from build123d import *

# Parameters (mm, degrees)
F1_DEPTH = 67.4566328526
F2_DEPTH = 6.2197912484
F4_DEPTH = 12.4627631158


with BuildPart() as f1:
    # F0 (on Right) → F1 (new body)
    with BuildSketch(Plane.YZ):
        Polygon((-5.8088302612, 34.2432931066), (0, 34.2432931066), (0, -34.2432931066), (-5.8088302612, -34.2432931066), (-5.8088302612, -37.9646643996), (76.7590999603, -37.9646643996), (76.7590999603, 37.9646643996), (-5.8088302612, 37.9646643996), align=None)
    extrude(amount=F1_DEPTH)

    # F2 (add): a face of the model
    f2_faces = [f1.faces().sort_by_distance(p)[0] for p in [
        (33.7283164263, 76.7590999603, 0),
    ]]
    extrude(f2_faces, amount=F2_DEPTH)

    # F3 (on face) → F4 (join)
    with BuildSketch(Plane(origin=(0, 82.9788912088, 0), x_dir=(-1, 0, 0), z_dir=(0, 1, 0))):
        with BuildLine():
            ThreePointArc((-38.3854716222, 0.9479600765), (-36.6591605512, 5.8587284108), (-37.6652367413, 10.9659396112))
            ThreePointArc((-37.6652367413, 10.9659396112), (-40.901393767, 22.4123427927), (-52.0788472287, 18.3432652315))
            ThreePointArc((-52.0788472287, 18.3432652315), (-65.9917417473, 22.0669934876), (-55.7989236075, 11.8914716641))
            Line((-55.7989236075, 11.8914716641), (-55.7989236075, 0))
            Line((-55.7989236075, 0), (-50.582356751, 6.5680034459))
            Line((-50.582356751, 6.5680034459), (-46.5246960521, 6.5680034459))
            ThreePointArc((-46.5246960521, 6.5680034459), (-44.599657899, 1.9303920858), (-44.8609884943, -3.0840787076))
            Line((-44.8609884943, -3.0840787076), (-38.3854716222, 0.9479600765))
        make_face()
    extrude(amount=F4_DEPTH)


solid = f1.part
Design review of the part built by this model. Coordinates are the model's own, in mm. A direction names the side the tool comes from. Round coordinates to 2 decimals unless told otherwise and drop trailing zeros. Write each loop counter-clockwise with the first axis right and the second up, starting at its lowest first coordinate (ties: lowest second). Pieces come first, ordered by that corner, then holes. Notation, with made-up numbers: M -12,61.5 L 36,61.5 A19 ccw 36,80.5 Z; hole C -39.5,12 d2. An arc over 180 degrees is marked long. One line per item, written item: value. Start each with the question number.
1. Take a section at C-C on z = -9. State the section outline as (x, y) points, then the cut area to 3 significant figures.
2. Draft analysis for pull direction Z (two halves, no side actions). For faces 5 (the face through (33, 0, 0)), 6 (the face through (55.799, 89, 6)), 7 (the face through (33, 38, -37.965)), 8 (the face through (33, -3, -34.243)), state which applies: pulls with the +Z half, pulls with the -Z half, needs draft (parallel to the pull), parting line crosses it, or undercut.
3. Take a section at A-A on x = 30.5. State the section outline as (y, z) points.
4. To check wall thickness, follow probe 1 along Y at (x, z) = (28, 31); probe 2 along Y at (x, z) = (59, 21); probe 3 along Z at (x, y) = (47, 86). State the ranges of each line that lie inside material, in increasing order. Write a range as from..to.
5. Clearance check with flat-ended pins moving along their axes: P1, Ø2, axis at x = 35.5, z = 1.5, coming from the +Y side; P2, Ø9.5, axis at y = 90.5, z = 4.5, coming from the +X side; P3, Ø5, axis at x = 56.5, z = 9, coming from the -Y side. State where each tip first meets the part, or that it passes through.
6. Take a section at B-B on y = 88. State the section outline as (x, z) points, then the cut area to 3 significant figures.
7. Take a section at D-D on x = 48.5. State the section outline as (y, z) points.
8. For faces 1 (the face through (36.665, 89.123, 5.785)), 2 (the face through (41.669, 89.123, -1.096)), 3 (the face through (44.61, 89.12, 2)), 4 (the face through (49, 89, 6.568)), list the 3-axis set-ups (+Z, -Z, +X, -X, +Y, -Y) from which the entire face can be reached by the end or side of a thin tool; tool diameter is ignored.
Computed:
1. outline: M 0,0 L 67.46,0 L 67.46,82.98 L 0,82.98 Z
1. area: 5,600 mm²
2. face 5: undercut
2. face 6: needs draft
2. face 7: pulls with the -Z half
2. face 8: undercut
3. outline: M -5.81,-37.96 L 82.98,-37.96 L 82.98,37.96 L -5.81,37.96 L -5.81,34.24 L 0,34.24 L 0,-34.24 L -5.81,-34.24 Z
4. probe 1: y = 0..82.98
4. probe 2: y = 0..95.44
4. probe 3: z = 6.57..22.94
5. P1: stops at y = 82.98
5. P2: stops at x = 55.8
5. P3: stops at y = 0
6. outline: M 37.67,10.97 A9.89 ccw 38.39,0.95 L 44.86,-3.08 A11.36 cw 46.52,6.57 L 50.58,6.57 L 55.8,0 L 55.8,11.89 A7.45 ccw long 52.08,18.34 A8.12 ccw long Z
6. area: 508 mm²
7. outline: M -5.81,-37.96 L 82.98,-37.96 L 82.98,6.57 L 95.44,6.57 L 95.44,22.31 L 82.98,22.31 L 82.98,37.96 L -5.81,37.96 L -5.81,34.24 L 0,34.24 L 0,-34.24 L -5.81,-34.24 Z
8. face 1: -X, +Y
8. face 2: -Z, -X, +Y
8. face 3: +Y
8. face 4: -Z, +Y
